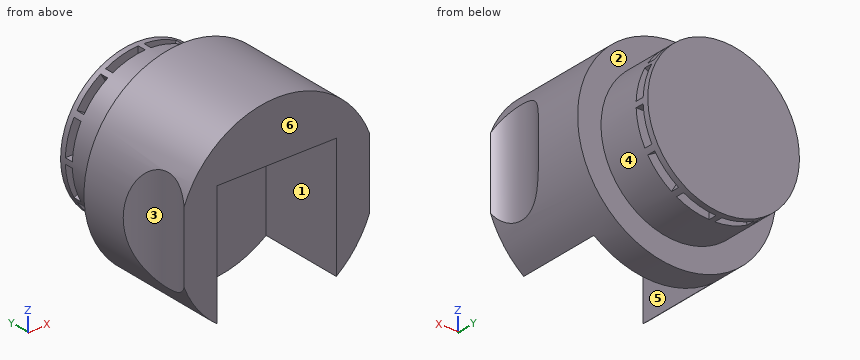
```python
from build123d import *

# Parameters (mm, degrees)
SKETCH_1_R               = 70
EXTRUDE_1_DEPTH          = 80
SKETCH_2_R               = 53.5
EXTRUDE_2_DEPTH          = 40
CUT_EXTRUDE_1_DEPTH      = 6
SKETCH_4_R               = 40
CUT_EXTRUDE_2_DEPTH      = 156.563491861
CUT_EXTRUDE_3_DEPTH      = 30
CUT_EXTRUDE_3_DEPTH_BACK = 156.563491951
SKETCH_5_W               = 84
SKETCH_5_H               = 120


with BuildPart() as part:
    # 草图1 → 凸台-拉伸1 (new body)
    with BuildSketch(Plane(origin=(0, 0, 0), x_dir=(1, 0, 0), z_dir=(0, 1, 0))):
        with Locations(Location((0, 0, 0), (0, 0, 270))):
            Circle(SKETCH_1_R)
    extrude(amount=EXTRUDE_1_DEPTH)

    # 草图2 → 凸台-拉伸2 (add)
    with BuildSketch(Plane(origin=(0, 80, 0), x_dir=(1, 0, 0), z_dir=(0, 1, 0))):
        with Locations(Location((0, 0, 0), (0, 0, 270))):
            Circle(SKETCH_2_R)
    extrude(amount=EXTRUDE_2_DEPTH)

    # 草图3 → 切除-拉伸1 (cut)
    with BuildSketch(Plane(origin=(0, 110, 0), x_dir=(1, 0, 0), z_dir=(0, 1, 0))):
        with BuildLine():
            ThreePointArc((-35.597687784, -18.242933548), (-38.637033052, -10.352761804), (-39.949968711, -2))
            Line((-39.949968711, -2), (-53.462603753, -2))
            ThreePointArc((-53.462603753, -2), (-51.677031706, -13.846818913), (-47.299973002, -24.999251069))
            Line((-47.299973002, -24.999251069), (-35.597687784, -18.242933548))
        make_face()
        with BuildLine():
            ThreePointArc((-39.949968711, 2), (-38.637033052, 10.352761804), (-35.597687784, 18.242933548))
            Line((-35.597687784, 18.242933548), (-47.299973002, 24.999251069))
            ThreePointArc((-47.299973002, 24.999251069), (-51.677031706, 13.846818913), (-53.462603753, 2))
            Line((-53.462603753, 2), (-39.949968711, 2))
        make_face()
        with BuildLine():
            ThreePointArc((-33.597687784, 21.707035163), (-28.284271247, 28.284271247), (-21.707035163, 33.597687784))
            Line((-21.707035163, 33.597687784), (-28.463352684, 45.299973002))
            ThreePointArc((-28.463352684, 45.299973002), (-37.830212793, 37.830212793), (-45.299973002, 28.463352684))
            Line((-45.299973002, 28.463352684), (-33.597687784, 21.707035163))
        make_face()
        with BuildLine():
            ThreePointArc((-18.242933548, 35.597687784), (-10.352761804, 38.637033052), (-2, 39.949968711))
            Line((-2, 39.949968711), (-2, 53.462603753))
            ThreePointArc((-2, 53.462603753), (-13.846818913, 51.677031706), (-24.999251069, 47.299973002))
            Line((-24.999251069, 47.299973002), (-18.242933548, 35.597687784))
        make_face()
        with BuildLine():
            Line((2, 53.462603753), (2, 39.949968711))
            ThreePointArc((2, 39.949968711), (10.352761804, 38.637033052), (18.242933548, 35.597687784))
            Line((18.242933548, 35.597687784), (24.999251069, 47.299973002))
            ThreePointArc((24.999251069, 47.299973002), (13.846818913, 51.677031706), (2, 53.462603753))
        make_face()
        with BuildLine():
            Line((28.463352684, 45.299973002), (21.707035163, 33.597687784))
            ThreePointArc((21.707035163, 33.597687784), (28.284271247, 28.284271247), (33.597687784, 21.707035163))
            Line((33.597687784, 21.707035163), (45.299973002, 28.463352684))
            ThreePointArc((45.299973002, 28.463352684), (37.830212793, 37.830212793), (28.463352684, 45.299973002))
        make_face()
        with BuildLine():
            Line((47.299973002, 24.999251069), (35.597687784, 18.242933548))
            ThreePointArc((35.597687784, 18.242933548), (38.637033052, 10.352761804), (39.949968711, 2))
            Line((39.949968711, 2), (53.462603753, 2))
            ThreePointArc((53.462603753, 2), (51.677031706, 13.846818913), (47.299973002, 24.999251069))
        make_face()
        with BuildLine():
            Line((53.462603753, -2), (39.949968711, -2))
            ThreePointArc((39.949968711, -2), (38.637033052, -10.352761804), (35.597687784, -18.242933548))
            Line((35.597687784, -18.242933548), (47.299973002, -24.999251069))
            ThreePointArc((47.299973002, -24.999251069), (51.677031706, -13.846818913), (53.462603753, -2))
        make_face()
        with BuildLine():
            Line((45.299973002, -28.463352684), (33.597687784, -21.707035163))
            ThreePointArc((33.597687784, -21.707035163), (28.284271247, -28.284271247), (21.707035163, -33.597687784))
            Line((21.707035163, -33.597687784), (28.463352684, -45.299973002))
            ThreePointArc((28.463352684, -45.299973002), (37.830212793, -37.830212793), (45.299973002, -28.463352684))
        make_face()
        with BuildLine():
            Line((24.999251069, -47.299973002), (18.242933548, -35.597687784))
            ThreePointArc((18.242933548, -35.597687784), (10.352761804, -38.637033052), (2, -39.949968711))
            Line((2, -39.949968711), (2, -53.462603753))
            ThreePointArc((2, -53.462603753), (13.846818913, -51.677031706), (24.999251069, -47.299973002))
        make_face()
        with BuildLine():
            ThreePointArc((-2, -39.949968711), (-10.352761804, -38.637033052), (-18.242933548, -35.597687784))
            Line((-18.242933548, -35.597687784), (-24.999251069, -47.299973002))
            ThreePointArc((-24.999251069, -47.299973002), (-13.846818913, -51.677031706), (-2, -53.462603753))
            Line((-2, -53.462603753), (-2, -39.949968711))
        make_face()
        with BuildLine():
            ThreePointArc((-21.707035163, -33.597687784), (-28.284271247, -28.284271247), (-33.597687784, -21.707035163))
            Line((-33.597687784, -21.707035163), (-45.299973002, -28.463352684))
            ThreePointArc((-45.299973002, -28.463352684), (-37.830212793, -37.830212793), (-28.463352684, -45.299973002))
            Line((-28.463352684, -45.299973002), (-21.707035163, -33.597687784))
        make_face()
    extrude(amount=CUT_EXTRUDE_1_DEPTH, mode=Mode.SUBTRACT)

    # 草图4 → 切除-拉伸2 (cut, symmetric)
    with BuildSketch(Plane.XY):
        with Locations((100, 20)):
            Circle(SKETCH_4_R)
    cut_extrude_2 = extrude(amount=CUT_EXTRUDE_2_DEPTH, both=True, mode=Mode.SUBTRACT)

    # 镜向1: 切除-拉伸2 across plane
    add(cut_extrude_2.mirror(Plane(origin=(0, 0, 0), x_dir=(0, 0, 1), z_dir=(1, 0, 0))), mode=Mode.SUBTRACT)

    # 草图5 → 切除-拉伸3 (cut, two sides: drawn at the far end of the back side and taken through both)
    with BuildSketch(Plane.XY.offset(-CUT_EXTRUDE_3_DEPTH_BACK)):
        Rectangle(SKETCH_5_W, SKETCH_5_H)
    extrude(amount=CUT_EXTRUDE_3_DEPTH + CUT_EXTRUDE_3_DEPTH_BACK, mode=Mode.SUBTRACT)


solid = part.part
```
Work out the finished part from the listing and answer in its coordinate system (mm). Face numbers are marked on the shaded views. A direction names the side the tool comes from. Coordinates: 2 decimals unless noted, no trailing zeros. Loops run counter-clockwise (first coordinate to the right, second up) from the corner with the lowest first, then second, coordinate; pieces in that order, holes last.
1) For a pull along X with two mould halves and no side action, classify the marked faces 1, 2 and 3 as +X half, -X half, draft (parallel to the pull), parting line (faces both ways), or undercut.
Results:
face 1: undercut
face 2: draft
face 3: -X half
2) Section A-A (x = 0) is taken. Give the vertices of the cut face in (y, z), plus the area to 3 significant figures.
Results:
outline: (0, 30) - (60, 30) - (60, -70) - (80, -70) - (80, -53.5) - (120, -53.5) - (120, 53.5) - (80, 53.5) - (80, 70) - (0, 70) - close
area: 9,480 mm2
3) Section B-B (z = 0) is taken. Give the vertices of the cut face in (x, y), plus the area to 3 significant figures.
Results:
outline: (-70, 46.46) arc R40 cw to (-65.36, 0) - (-42, 0) - (-42, 60) - (42, 60) - (42, 0) - (65.36, 0) arc R40 cw to (70, 46.46) - (70, 80) - (53.5, 80) - (53.5, 120) - (-53.5, 120) - (-53.5, 80) - (-70, 80) - close
area: 9,750 mm2
4) Flat-ended cylindrical pins translate along their axes: pin 1 (8 mm diameter, centred on y = 14.5, z = 47.5, fed in from +X); pin 2 (9 mm diameter, centred on x = -8, z = -44.5, fed in from -Y); pin 3 (1 mm diameter, centred on y = 28.5, z = 43.5, fed in from +X). Find the tip coordinate at first contact, or state that the pin passes through.
Results:
pin 1: stops at x = 54.84
pin 2: stops at y = 60
pin 3: stops at x = 55.24
5) Section C-C (y = 65) is taken. Give the vertices of the cut face in (x, z), plus the area to 3 significant figures.
Results:
outline: circle Ø140 at (0, 0)
area: 15,400 mm2
6) Section D-D (z = -49.5) is taken. Give the vertices of the cut face in (x, y), plus the area to 3 significant figures.
Results:
outline: (-49.49, 0) - (-42, 0) - (-42, 60) - (42, 60) - (42, 0) - (49.49, 0) - (49.49, 80) - (20.3, 80) - (20.3, 110) - (2, 110) - (2, 116) - (20.3, 116) - (20.3, 120) - (-20.3, 120) - (-20.3, 116) - (-2, 116) - (-2, 110) - (-20.3, 110) - (-20.3, 80) - (-49.49, 80) - close
area: 4,280 mm2
7) Consider probe 1 along X at (y, z) = (59, -33.5); probe 2 along Y at (x, z) = (-27, -57.5); probe 3 along X at (y, z) = (45, 27). Determine where each line is inside the solid, lowest interval first.
Results:
probe 1: x = -61.46 to -42, 42 to 61.46
probe 2: y = 60 to 80
probe 3: x = -64.58 to -42, 42 to 64.58
8) For the marked faces 4, 5 and 6, determine the directions among +Z, -Z, +X, -X, +Y, -Y from which every point of the face is accessible in a straight line to the end or side of a thin tool.
Results:
face 4: +Y
face 5: -Z, -Y
face 6: +Z, -Z, +X, -X, -Y
